Geometry check sheet. Reference: drawing and pictorial views, mm from the part's lowest x, y, z. Coordinates: 2 decimals unless noted, no trailing zeros. Loops run counter-clockwise (first coordinate to the right, second up) from the corner with the lowest first, then second, coordinate; pieces in that order, holes last. Notation, with made-up numbers: (51.25, 31) -> (108.25, 31) arc R14 cw to (108.25, 52) -> close; hole circle Ø7 at (40, 32.5). An arc over 180 degrees is marked (long way). Use one line per item in the form item = value.
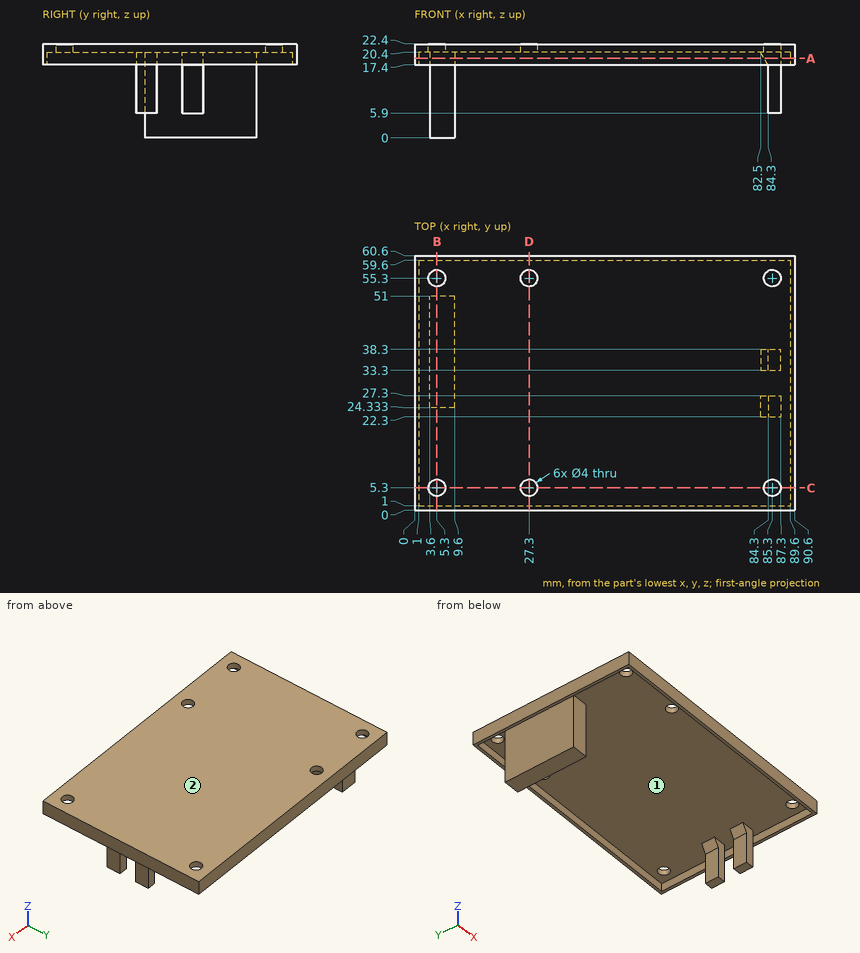
(1) Section check A-A, the plane z = 19. Record the boundary of the cut face in (x, y), plus the area to 3 significant figures.
Established:
outline = (0, 0) -> (90.6, 0) -> (90.6, 60.6) -> (0, 60.6) -> close; (3.6, 24.33) -> (9.6, 24.33) -> (9.6, 51) -> (3.6, 51) -> close; (83.34, 22.3) -> (87.3, 22.3) -> (87.3, 27.3) -> (83.34, 27.3) -> close; (83.34, 33.3) -> (87.3, 33.3) -> (87.3, 38.3) -> (83.34, 38.3) -> close; hole (1, 1) -> (89.6, 1) -> (89.6, 59.6) -> (1, 59.6) -> close
area = 498 mm²
(2) Section check C-C, the plane y = 5.3. Record the boundary of the cut face in (x, z).
Established:
outline = (0, 17.4) -> (1, 17.4) -> (1, 20.4) -> (3.3, 20.4) -> (3.3, 22.4) -> (0, 22.4) -> close; (7.3, 20.4) -> (25.3, 20.4) -> (25.3, 22.4) -> (7.3, 22.4) -> close; (29.3, 20.4) -> (83.3, 20.4) -> (83.3, 22.4) -> (29.3, 22.4) -> close; (87.3, 20.4) -> (89.6, 20.4) -> (89.6, 17.4) -> (90.6, 17.4) -> (90.6, 22.4) -> (87.3, 22.4) -> close
(3) Section check B-B, the plane x = 5.3. Record the boundary of the cut face in (y, z), plus the area to 3 significant figures.
Established:
outline = (0, 17.4) -> (1, 17.4) -> (1, 20.4) -> (3.3, 20.4) -> (3.3, 22.4) -> (0, 22.4) -> close; (7.3, 20.4) -> (24.33, 20.4) -> (24.33, 0) -> (51, 0) -> (51, 20.4) -> (53.3, 20.4) -> (53.3, 22.4) -> (7.3, 22.4) -> close; (57.3, 20.4) -> (59.6, 20.4) -> (59.6, 17.4) -> (60.6, 17.4) -> (60.6, 22.4) -> (57.3, 22.4) -> close
area = 655 mm²
(4) Section check D-D, the plane x = 27.3. Record the boundary of the cut face in (y, z), plus the area to 3 significant figures.
Established:
outline = (0, 17.4) -> (1, 17.4) -> (1, 20.4) -> (3.3, 20.4) -> (3.3, 22.4) -> (0, 22.4) -> close; (7.3, 20.4) -> (53.3, 20.4) -> (53.3, 22.4) -> (7.3, 22.4) -> close; (57.3, 20.4) -> (59.6, 20.4) -> (59.6, 17.4) -> (60.6, 17.4) -> (60.6, 22.4) -> (57.3, 22.4) -> close
area = 111 mm²
(5) Scan lines: line 1 along Y through (x, z) = (85.3, 21.65); line 2 along Z through (x, y) = (58, 15); line 3 along Y through (x, z) = (5, 1.25). Record each from-to range of solid material in increasing order.
Established:
line_1 = 0 to 3.3, 7.3 to 53.3, 57.3 to 60.6
line_2 = 20.4 to 22.4
line_3 = 24.33 to 51
(6) Mould release check, pull along Y, two halves, no side actions. Record for the marked faces 1 and 2: +Y half, -Y half, draft (parallel to the pull), parting line (faces both ways), or undercut.
Established:
face_1 = undercut
face_2 = draft
(7) Go/stop test with flat-tipped pins: P1, Ø12, axis at y = 12.5, z = 8, coming from the -X side; P2, Ø4, axis at y = 26, z = 10, coming from the -X side; P3, Ø1.5, axis at x = 86.5, y = 24.5, coming from the -Z side; P4, Ø6.5, axis at x = 7, z = 6, coming from the -Y side. Record where each tip stops, or that it passes through.
Established:
P1 = through
P2 = 3.6
P3 = 5.9
P4 = 24.33
